Part model, mm, in its own coordinate system. Round coordinates to 2 decimals unless told otherwise and drop trailing zeros. Write each loop counter-clockwise with the first axis right and the second up, starting at its lowest first coordinate (ties: lowest second). Pieces come first, ordered by that corner, then holes.
1) Saw through at A-A on z = 0.45. Write the cut outline in (x, y), and give its area (3 significant figures).
2) Saw through at B-B on x = 134.5. Write the cut outline in (y, z), and give its area (3 significant figures).
3) Drill centre lines: L1, parallel to X at y = -97, z = 1.05; L2, parallel to Y at x = 71.5, z = 1.45; L3, parallel to Y at x = 191, z = 1.1. Where is each one in solid material? Low to high.
4) Flat gauge pins, fed straight in: pin 1 (1.5 mm diameter, centred on x = -35.5, z = 2.5, fed in from -Y); pin 2 (1.4 mm diameter, centred on y = -101.5, z = 2, fed in from +X). Where does each tip first touch, or does it go through?
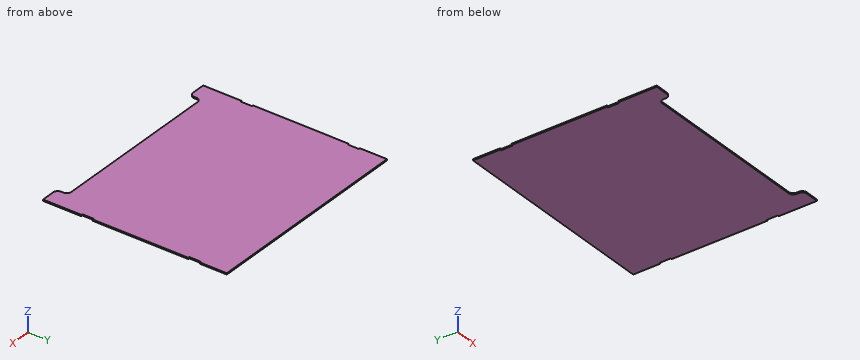
```python
from build123d import *

# Parameters (mm, degrees)
BOSS_EXTRUDE1_DEPTH = 2.9


with BuildPart() as part:
    # Sketch1 → Boss-Extrude1 (new body)
    with BuildSketch(Plane.XY):
        with BuildLine():
            Line((206.1, -203.2), (236.1, -203.2))
            Line((236.1, -203.2), (236.1, -118.2))
            Line((236.1, -118.2), (233.2, -118.2))
            Line((233.2, -118.2), (233.2, -93.2))
            Line((233.2, -93.2), (236.1, -93.2))
            Line((236.1, -93.2), (236.1, 118.2))
            Line((236.1, 118.2), (233.2, 118.2))
            Line((233.2, 118.2), (233.2, 143.2))
            Line((233.2, 143.2), (236.1, 143.2))
            Line((236.1, 143.2), (236.1, 203.2))
            Line((236.1, 203.2), (-236.1, 203.2))
            Line((-236.1, 203.2), (-236.1, 143.2))
            Line((-236.1, 143.2), (-233.2, 143.2))
            Line((-233.2, 143.2), (-233.2, 118.2))
            Line((-233.2, 118.2), (-236.1, 118.2))
            Line((-236.1, 118.2), (-236.1, -93.2))
            Line((-236.1, -93.2), (-233.2, -93.2))
            Line((-233.2, -93.2), (-233.2, -118.2))
            Line((-233.2, -118.2), (-236.1, -118.2))
            Line((-236.1, -118.2), (-236.1, -203.2))
            Line((-236.1, -203.2), (-206.1, -203.2))
            ThreePointArc((-206.1, -203.2), (-199.028932188, -200.271067812), (-196.1, -193.2))
            Line((-196.1, -193.2), (-196.1, -188.2))
            ThreePointArc((-196.1, -188.2), (-193.171067812, -181.128932188), (-186.1, -178.2))
            Line((-186.1, -178.2), (186.1, -178.2))
            ThreePointArc((186.1, -178.2), (193.171067812, -181.128932188), (196.1, -188.2))
            Line((196.1, -188.2), (196.1, -193.2))
            ThreePointArc((196.1, -193.2), (199.028932188, -200.271067812), (206.1, -203.2))
        make_face()
    extrude(amount=BOSS_EXTRUDE1_DEPTH)


solid = part.part
```
Completed:
1. outline: (-236.1, -203.2) - (-206.1, -203.2) arc R10 ccw to (-196.1, -193.2) - (-196.1, -188.2) arc R10 cw to (-186.1, -178.2) - (186.1, -178.2) arc R10 cw to (196.1, -188.2) - (196.1, -193.2) arc R10 ccw to (206.1, -203.2) - (236.1, -203.2) - (236.1, -118.2) - (233.2, -118.2) - (233.2, -93.2) - (236.1, -93.2) - (236.1, 118.2) - (233.2, 118.2) - (233.2, 143.2) - (236.1, 143.2) - (236.1, 203.2) - (-236.1, 203.2) - (-236.1, 143.2) - (-233.2, 143.2) - (-233.2, 118.2) - (-236.1, 118.2) - (-236.1, -93.2) - (-233.2, -93.2) - (-233.2, -118.2) - (-236.1, -118.2) - close
1. area: 182,000 mm2
2. outline: (-178.2, 0) - (203.2, 0) - (203.2, 2.9) - (-178.2, 2.9) - close
2. area: 1,110 mm2
3. L1: x = -233.2 to 233.2
3. L2: y = -178.2 to 203.2
3. L3: y = -179.48 to 203.2
4. pin 1: stops at y = -178.2
4. pin 2: stops at x = 233.2
